```python
from build123d import *

# Parameters (mm, degrees)
F0_R      = 15
F1_DEPTH  = 80
F2_R      = 18
F3_DEPTH  = 50
F6_D      = 6.35
F8_D      = 21
F8_DEPTH  = 45
F8_TIP    = 6.3090364998
F10_D     = 22.4
F10_DEPTH = 6
F10_TIP   = 6.7296389331
F11_SIZE  = 2


with BuildPart() as f1:
    # F0 (on Top) → F1 (new body)
    with BuildSketch(Plane.XY):
        Circle(F0_R)
    extrude(amount=F1_DEPTH)

    # F2 (on Top) → F3 (join)
    with BuildSketch(Plane.XY):
        Circle(F2_R)
    extrude(amount=F3_DEPTH)

    # F6 (through all)
    with Locations(Plane.XY.offset(80)):
        with Locations((0, 0)):
            Hole(F6_D / 2)

    # F8
    with Locations(Plane.XY.offset(80)):
        with Locations((0, 0)):
            Hole(F8_D / 2, depth=F8_DEPTH)
            with Locations((0, 0, -(F8_DEPTH + F8_TIP / 2))):  # 118° drill point
                Cone(0, F8_D / 2, F8_TIP, mode=Mode.SUBTRACT)

    # F10
    with Locations(Plane.XY.offset(80)):
        with Locations((0, 0)):
            Hole(F10_D / 2, depth=F10_DEPTH)
            with Locations((0, 0, -(F10_DEPTH + F10_TIP / 2))):  # 118° drill point
                Cone(0, F10_D / 2, F10_TIP, mode=Mode.SUBTRACT)

    # F11
    f11_edges = [f1.edges().sort_by_distance(p)[0] for p in [
        (-15, 0, 80),
    ]]
    chamfer(f11_edges, length=F11_SIZE)


solid = f1.part
```
For this review, take the finished solid that the model builds, in its own axes (mm). A direction names the side the tool comes from. Coordinates: 2 decimals unless noted, no trailing zeros. Order: outer loops, then holes, each group sorted by start corner. A loop starts at its lowest first (then second) coordinate and runs counter-clockwise, first axis right, second up. Notation, with made-up numbers: (-8.5, 2.25) -> (19.5, 2.25) arc R17 ccw to (19.5, 16.25) -> close; hole circle Ø11 at (34, 19). An arc over 180 degrees is marked (long way). Use CSV: the item, a comma, the result in double quotes. Start each with the question number.
Item 1: For faces 1 (the face through (4, 11, 80)), 2 (the face through (11.19, 0.49, 76.96)), list the 3-axis set-ups (+Z, -Z, +X, -X, +Y, -Y) from which the entire face can be reached by the end or side of a thin tool; tool diameter is ignored.
Item 2: Draft analysis for pull direction X (two halves, no side actions). For faces 3 (the face through (-14.985, 0.66, 63.804)), 4 (the face through (-10, 3.2, 54)), 5 (the face through (-4, 15, 50)), state which applies: pulls with the +X half, pulls with the -X half, needs draft (parallel to the pull), parting line crosses it, or undercut.
Item 3: Wall thickness on probe 1 along X at (y, z) = (0, 76.85); probe 2 along Y at (x, z) = (0, 46); probe 3 along Y at (x, z) = (0, 11.5) (3 decimals): over which ranges is each line inside the solid? List them lowest first.
Item 4: We need section A-A, the plane y = 0. Give the boundary of the cut face in (x, z) (3 decimals).
Item 5: We need section D-D, the plane z = 60. Give the boundary of the cut face in (x, y).
Item 6: We need section C-C, the plane z = 15.5. Give the boundary of the cut face in (x, y) (3 decimals), then the cut area to 3 significant figures.
Item 7: Insertion check: pin 1 (2 mm diameter, centred on y = -0.5, z = 25.5, fed in from +X); pin 2 (12 mm diameter, centred on x = 9, z = 42, fed in from +Y); pin 3 (2 mm diameter, centred on x = 6, y = 5, fed in from +Z); pin 4 (5 mm diameter, centred on x = 7, z = 14, fed in from -Y). Each pin has a flat end and moves straight along its axis. Give the tip position at first contact, or say it passes through.
Derived:
1,face 1,"+Z, +X, -X, +Y, -Y"
1,face 2,"+Z"
2,face 3,"parting line crosses it"
2,face 4,"undercut"
2,face 5,"needs draft"
3,probe 1,"x = -15 to -11.2, 11.2 to 15"
3,probe 2,"y = -18 to -10.5, 10.5 to 18"
3,probe 3,"y = -18 to -3.175, 3.175 to 18"
4,outline,"(-18, 0) -> (-3.175, 0) -> (-3.175, 30.599) -> (-10.5, 35) -> (-10.5, 73.579) -> (-11.2, 74) -> (-11.2, 80) -> (-13, 80) -> (-15, 78) -> (-15, 50) -> (-18, 50) -> close; (3.175, 0) -> (18, 0) -> (18, 50) -> (15, 50) -> (15, 78) -> (13, 80) -> (11.2, 80) -> (11.2, 74) -> (10.5, 73.579) -> (10.5, 35) -> (3.175, 30.599) -> close"
5,outline,"circle Ø30 at (0, 0); hole circle Ø21 at (0, 0)"
6,outline,"circle Ø36 at (0, 0); hole circle Ø6.35 at (0, 0)"
6,area,"986 mm^2"
7,pin 1,"stops at x = 18"
7,pin 2,"stops at y = 17.75"
7,pin 3,"stops at z = 33.98"
7,pin 4,"stops at y = -17.43"
